Design review of the part built by this model. Coordinates are the model's own, in mm. Give positions to 0.01 mm unless a question says otherwise; leave off trailing zeros. Order: outer loops, then holes, each group sorted by start corner. A loop starts at its lowest first (then second) coordinate and runs counter-clockwise, first axis right, second up.
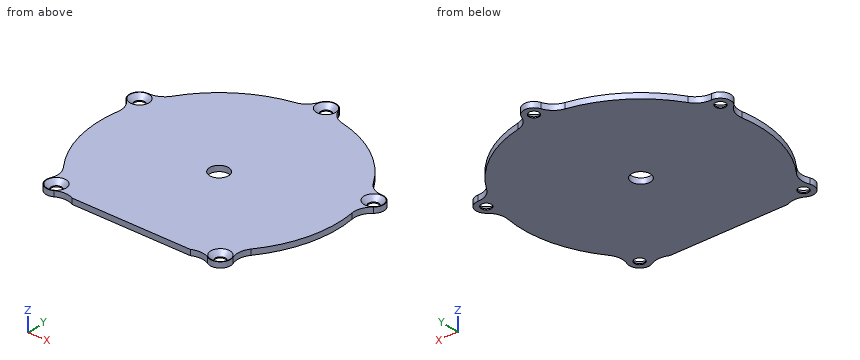
```python
from build123d import *

# Parameters (mm, degrees)
BOSS_EXTRUDE1_DEPTH                          = 3
CSK_FOR_M5_COUNTERSUNK_FLAT_HEAD_SCR_2_COUNT = 2
CSK_FOR_M5_COUNTERSUNK_FLAT_HEAD_SCR_2_PITCH = 76.842304832
CSK_FOR_M5_COUNTERSUNK_FLAT_HEAD_SCR_3_COUNT = 2
CSK_FOR_M5_COUNTERSUNK_FLAT_HEAD_SCR_3_PITCH = 126.274488939
CSK_FOR_M5_COUNTERSUNK_FLAT_HEAD_SCR_4_COUNT = 2
CSK_FOR_M5_COUNTERSUNK_FLAT_HEAD_SCR_4_PITCH = 130.663789522
CSK_FOR_M5_COUNTERSUNK_FLAT_HEAD_SCR_5_COUNT = 2
CSK_FOR_M5_COUNTERSUNK_FLAT_HEAD_SCR_5_PITCH = 76.842304832
SKETCH7_R                                    = 5.1
CUT_EXTRUDE1_DEPTH                           = 101.176561813


with BuildPart() as part:
    # Sketch1 → Boss-Extrude1 (new body)
    with BuildSketch(Plane.XY):
        with BuildLine():
            Line((-31.845730134, -55.405913397), (0, -55.405913397))
            Line((0, -55.405913397), (31.845730134, -55.405913397))
            ThreePointArc((31.845730134, -55.405913397), (36.683914759, -54.28538737), (41.464515841, -55.630549937))
            ThreePointArc((41.464515841, -55.630549937), (47.829334185, -55.023876328), (49.319655375, -48.806327923))
            ThreePointArc((49.319655375, -48.806327923), (48.678987264, -43.702284601), (50.66032125, -38.955071786))
            ThreePointArc((50.66032125, -38.955071786), (61.939586577, -15.730651027), (63.108911007, 10.061367629))
            ThreePointArc((63.108911007, 10.061367629), (63.632854976, 15.178710356), (66.631324059, 19.35853057))
            ThreePointArc((66.631324059, 19.35853057), (68.28894151, 25.532189009), (62.987637378, 29.104013283))
            ThreePointArc((62.987637378, 29.104013283), (57.982455244, 30.291390926), (54.229750811, 33.809760336))
            ThreePointArc((54.229750811, 33.809760336), (36.426163747, 52.508098059), (12.677003214, 62.635927043))
            ThreePointArc((12.677003214, 62.635927043), (8.067219644, 64.918821983), (5.202184299, 69.191208475))
            ThreePointArc((5.202184299, 69.191208475), (0, 72.905913397), (-5.202184299, 69.191208475))
            ThreePointArc((-5.202184299, 69.191208475), (-8.067219644, 64.918821983), (-12.677003214, 62.635927043))
            ThreePointArc((-12.677003214, 62.635927043), (-36.426163747, 52.508098059), (-54.229750811, 33.809760336))
            ThreePointArc((-54.229750811, 33.809760336), (-57.982455244, 30.291390926), (-62.987637378, 29.104013283))
            ThreePointArc((-62.987637378, 29.104013283), (-68.28894151, 25.532189009), (-66.631324059, 19.35853057))
            ThreePointArc((-66.631324059, 19.35853057), (-63.632854976, 15.178710356), (-63.108911007, 10.061367629))
            ThreePointArc((-63.108911007, 10.061367629), (-61.939586577, -15.730651027), (-50.66032125, -38.955071786))
            ThreePointArc((-50.66032125, -38.955071786), (-48.678987264, -43.702284601), (-49.319655375, -48.806327923))
            ThreePointArc((-49.319655375, -48.806327923), (-47.829334185, -55.023876328), (-41.464515841, -55.630549937))
            ThreePointArc((-41.464515841, -55.630549937), (-36.683914759, -54.28538737), (-31.845730134, -55.405913397))
        make_face()
    extrude(amount=BOSS_EXTRUDE1_DEPTH)

    # Sketch3 → CSK for M5 Countersunk Flat Head Screw1 (revolve, cut)
    with BuildSketch(Plane(origin=(-63.13724447, 23.606048412, 3), x_dir=(0, -1, 0), z_dir=(1, 0, 0))):
        Polygon((0, 0), (0, 3), (2.75, 3), (2.75, 2.45), (5.2, 0), align=None)
    csk_for_m5_countersunk_flat_head_screw1 = revolve(axis=Axis((-63.13724447, 23.606048412, 9.35), (0, 0, -1)), mode=Mode.SUBTRACT)

    # CSK for M5 Countersunk Flat Head Scr 2: CSK for M5 Countersunk Flat Head Screw1 ×2
    with Locations(*[Vector(0.8216469379421629, 0.5699967625963042, 0) * (i * CSK_FOR_M5_COUNTERSUNK_FLAT_HEAD_SCR_2_PITCH) for i in range(1, CSK_FOR_M5_COUNTERSUNK_FLAT_HEAD_SCR_2_COUNT)]):
        add(csk_for_m5_countersunk_flat_head_screw1, mode=Mode.SUBTRACT)

    # CSK for M5 Countersunk Flat Head Scr 3: CSK for M5 Countersunk Flat Head Screw1 ×2
    with Locations(*[(i * CSK_FOR_M5_COUNTERSUNK_FLAT_HEAD_SCR_3_PITCH, 0, 0) for i in range(1, CSK_FOR_M5_COUNTERSUNK_FLAT_HEAD_SCR_3_COUNT)]):
        add(csk_for_m5_countersunk_flat_head_screw1, mode=Mode.SUBTRACT)

    # CSK for M5 Countersunk Flat Head Scr 4: CSK for M5 Countersunk Flat Head Screw1 ×2
    with Locations(*[Vector(0.8216469379421629, -0.5699967625963043, 0) * (i * CSK_FOR_M5_COUNTERSUNK_FLAT_HEAD_SCR_4_PITCH) for i in range(1, CSK_FOR_M5_COUNTERSUNK_FLAT_HEAD_SCR_4_COUNT)]):
        add(csk_for_m5_countersunk_flat_head_screw1, mode=Mode.SUBTRACT)

    # CSK for M5 Countersunk Flat Head Scr 5: CSK for M5 Countersunk Flat Head Screw1 ×2
    with Locations(*[Vector(0.24615329302899694, -0.9692309097067534, 0) * (i * CSK_FOR_M5_COUNTERSUNK_FLAT_HEAD_SCR_5_PITCH) for i in range(1, CSK_FOR_M5_COUNTERSUNK_FLAT_HEAD_SCR_5_COUNT)]):
        add(csk_for_m5_countersunk_flat_head_screw1, mode=Mode.SUBTRACT)

    # Sketch7 → Cut-Extrude1 (cut, through all)
    with BuildSketch(Plane.XY.offset(3)):
        Circle(SKETCH7_R)
    extrude(amount=-CUT_EXTRUDE1_DEPTH, mode=Mode.SUBTRACT)


solid = part.part
```
1. For line 1 along Y through (x, z) = (0, 0.1); line 2 along Y through (x, z) = (2, 0.9); line 3 along Y through (x, z) = (14.5, 0.6), list the stretches that pass through material, from the lowest coordinate up.
Recorded:
line 1: y = -55.41 to -5.1, 5.1 to 64.66, 70.16 to 72.91
line 2: y = -55.41 to -4.69, 4.69 to 65.04, 69.77 to 72.53
line 3: y = -55.41 to 62.24
2. Take a section at B-B (x = 0). State the section outline as (y, z) points.
Recorded:
outline: (-55.41, 0) - (-5.1, 0) - (-5.1, 3) - (-55.41, 3) - close; (5.1, 0) - (64.66, 0) - (64.66, 0.55) - (62.21, 3) - (5.1, 3) - close; (70.16, 0) - (72.91, 0) - (72.91, 3) - (72.61, 3) - (70.16, 0.55) - close
3. Take a section at D-D (x = -52.5). State the section outline as (y, z) points.
Recorded:
outline: (-36.44, 0) - (36.44, 0) - (36.44, 3) - (-36.44, 3) - close
4. Take a section at C-C (z = 1.45). State the section outline as (x, y) points.
Recorded:
outline: (-66.63, 19.36) arc R10 cw to (-63.11, 10.06) arc R63.91 ccw to (-50.66, -38.96) arc R10 cw to (-49.32, -48.81) arc R5.5 ccw to (-41.46, -55.63) arc R10 cw to (-31.85, -55.41) - (31.85, -55.41) arc R10 cw to (41.46, -55.63) arc R5.5 ccw to (49.32, -48.81) arc R10 cw to (50.66, -38.96) arc R63.91 ccw to (63.11, 10.06) arc R10 cw to (66.63, 19.36) arc R5.5 ccw to (62.99, 29.1) arc R10 cw to (54.23, 33.81) arc R63.91 ccw to (12.68, 62.64) arc R10 cw to (5.2, 69.19) arc R5.5 ccw to (-5.2, 69.19) arc R10 cw to (-12.68, 62.64) arc R63.91 ccw to (-54.23, 33.81) arc R10 cw to (-62.99, 29.1) arc R5.5 ccw to start; hole circle Ø7.3 at (-63.14, 23.61); hole circle Ø7.3 at (-44.22, -50.87); hole circle Ø10.2 at (0, 0); hole circle Ø7.3 at (0, 67.41); hole circle Ø7.3 at (44.22, -50.87); hole circle Ø7.3 at (63.14, 23.61)
5. Take a section at A-A (y = 0). State the section outline as (x, z) points.
Recorded:
outline: (-63.91, 0) - (-5.1, 0) - (-5.1, 3) - (-63.91, 3) - close; (5.1, 0) - (63.91, 0) - (63.91, 3) - (5.1, 3) - close
6. For pin 1 (9 mm diameter, centred on x = -63.14, y = 23.61, fed in from +Z); pin 2 (3.5 mm diameter, centred on x = -44.22, y = -50.87, fed in from -Z); pin 3 (1 mm diameter, centred on y = 20, z = 1, fed in from -X); pin 4 (1.5 mm diameter, centred on x = 53.5, z = 1.5, fed in from +Y), all flat-tipped, find the tip position at first contact; note any pin that passes through.
Recorded:
pin 1: stops at z = 2.3
pin 2: passes through
pin 3: stops at x = -67.68
pin 4: stops at y = 36.07
